Design review of the part built by this model. Coordinates are the model's own, in mm. A direction names the side the tool comes from. Round coordinates to 2 decimals unless told otherwise and drop trailing zeros. Loops run counter-clockwise (first coordinate to the right, second up) from the corner with the lowest first, then second, coordinate; pieces in that order, holes last. Notation, with made-up numbers: (46.5, 32) -> (71.5, 32) arc R17 ccw to (71.5, 61) -> close; hole circle Ø11 at (69, -30.5). An arc over 180 degrees is marked (long way). Write each question's results on one line, items separated by ' | '. Start each with the question number.
from build123d import *

# Parameters (mm, degrees)
SKETCH1_W           = 20
SKETCH1_H           = 32
SKETCH1_W_2         = 100
SKETCH1_H_2         = 24
BOSS_EXTRUDE1_DEPTH = 20
BOSS_EXTRUDE2_START = 20
SKETCH1_3_W         = 20
SKETCH1_3_H         = 32
BOSS_EXTRUDE2_DEPTH = 10
BOSS_EXTRUDE3_START = 20
SKETCH1_5_W         = 100
SKETCH1_5_H         = 24
SKETCH1_5_H_2       = 52
SKETCH1_5_R         = 22.5
BOSS_EXTRUDE3_DEPTH = 10


with BuildPart() as part:
    # Sketch1 → Boss-Extrude1 (new body)
    with BuildSketch(Plane(origin=(0, 0, 0), x_dir=(1, 0, 0), z_dir=(0, 1, 0))):
        Polygon((50, -50), (-50, -50), (-50, -26), (-58, -26), (-58, -58), (77, -58), (77, -26), (50, -26), align=None)
        Polygon((-58, 26), (-50, 26), (-50, 50), (50, 50), (50, 26), (77, 26), (77, 58), (-58, 58), align=None)
        with Locations((87, -42)):
            Rectangle(SKETCH1_W, SKETCH1_H)
        with Locations((87, 42)):
            Rectangle(SKETCH1_W, SKETCH1_H)
        with Locations((0, -38)):
            Rectangle(SKETCH1_W_2, SKETCH1_H_2)
        with Locations((0, 38)):
            Rectangle(SKETCH1_W_2, SKETCH1_H_2)
    extrude(amount=BOSS_EXTRUDE1_DEPTH)

    # Sketch1<3> → Boss-Extrude2 (add)
    with BuildSketch(Plane(origin=(0, 0, 0), x_dir=(1, 0, 0), z_dir=(0, 1, 0)).offset(BOSS_EXTRUDE2_START)):
        with Locations((87, -42)):
            Rectangle(SKETCH1_3_W, SKETCH1_3_H)
        with Locations((87, 42)):
            Rectangle(SKETCH1_3_W, SKETCH1_3_H)
    extrude(amount=BOSS_EXTRUDE2_DEPTH)

    # Sketch1<5> → Boss-Extrude3 (add)
    # profile 1 of 3: a face of its own
    with BuildSketch(Plane(origin=(0, 0, 0), x_dir=(1, 0, 0), z_dir=(0, 1, 0)).offset(BOSS_EXTRUDE3_START)):
        with Locations((0, -38)):
            Rectangle(SKETCH1_5_W, SKETCH1_5_H)
    # profile 2 of 3: a face of its own
    with BuildSketch(Plane(origin=(0, 0, 0), x_dir=(1, 0, 0), z_dir=(0, 1, 0)).offset(BOSS_EXTRUDE3_START)):
        Rectangle(SKETCH1_5_W, SKETCH1_5_H_2)
        with Locations(Location((0, 0, 0), (0, 0, 270))):
            Circle(SKETCH1_5_R, mode=Mode.SUBTRACT)
    # profile 3 of 3: a face of its own
    with BuildSketch(Plane(origin=(0, 0, 0), x_dir=(1, 0, 0), z_dir=(0, 1, 0)).offset(BOSS_EXTRUDE3_START)):
        with Locations((0, 38)):
            Rectangle(SKETCH1_5_W, SKETCH1_5_H)
    extrude(amount=BOSS_EXTRUDE3_DEPTH)


solid = part.part
1) Take a section at B-B (z = 0). Write out the cut boundary in (x, y), plus the area to 3 significant figures.
2) Take a section at D-D (x = -29.5). Write out the cut boundary in (y, z).
3) Take a section at A-A (y = 3.25). Write out the cut boundary in (x, z), plus the area to 3 significant figures.
4) The part is to be moulded in two halves that separate along X. For faces 1 (the face through (24, 20, 52)), 2 (the face through (87, 30, 42)), 3 (the face through (-58, 10, -42)), say which applies: +X half, -X half, draft (parallel to the pull), parting line (faces both ways), or undercut.
5) Take a section at C-C (x = 0). Write out the cut boundary in (y, z).
6) For faces 4 (the face through (-23, 20, 0)), 5 (the face through (77, 25, 42)), 6 (the face through (-1, 25, 50)), list the 3-axis set-ups (+Z, -Z, +X, -X, +Y, -Y) from which the entire face can be reached by the end or side of a thin tool; tool diameter is ignored.
7) Insertion check: pin 1 (8 mm diameter, centred on x = 39, z = 12, fed in from -Y); pin 2 (8 mm diameter, centred on x = -23.5, y = 26.5, fed in from +Z); pin 3 (3 mm diameter, centred on y = 24, z = 17, fed in from +X); pin 4 (2 mm diameter, centred on y = 17.5, z = 1, fed in from +X). Each pin has a flat end and moves straight along its axis. Give the tip position at first contact, or say it passes through.
8) To check wall thickness, follow line 1 (Z direction, x = -12, y = 13.75); line 2 (X direction, y = 27.25, z = 0); line 3 (Y direction, x = -48, z = -23). State the ranges of each line that lie inside material, in increasing order. Write a range as from..to.
Geometry check:
1) outline: (-50, 20) -> (-22.5, 20) -> (-22.5, 30) -> (-50, 30) -> close; (22.5, 20) -> (50, 20) -> (50, 30) -> (22.5, 30) -> close | area: 550 mm^2
2) outline: (0, -58) -> (20, -58) -> (20, -50) -> (30, -50) -> (30, 50) -> (20, 50) -> (20, 58) -> (0, 58) -> (0, 26) -> (20, 26) -> (20, -26) -> (0, -26) -> close
3) outline: (-58, -58) -> (97, -58) -> (97, -26) -> (-58, -26) -> close; (-58, 26) -> (97, 26) -> (97, 58) -> (-58, 58) -> close | area: 9,920 mm^2
4) face 1: undercut | face 2: draft | face 3: -X half
5) outline: (0, -58) -> (20, -58) -> (20, -50) -> (30, -50) -> (30, -22.5) -> (20, -22.5) -> (20, -26) -> (0, -26) -> close; (0, 26) -> (20, 26) -> (20, 22.5) -> (30, 22.5) -> (30, 50) -> (20, 50) -> (20, 58) -> (0, 58) -> close
6) face 4: +X, -X, -Y | face 5: +Z, -Z, +Y | face 6: +Z, -X, +Y
7) pin 1: stops at y = 20 | pin 2: stops at z = 50 | pin 3: stops at x = 50 | pin 4: passes through
8) line 1: z = -58..-26, 26..58 | line 2: x = -50..-22.5, 22.5..50 | line 3: y = 20..30
